```python
from build123d import *

# Parameters (mm, degrees)
SKETCH1_W           = 60
SKETCH1_H           = 35
BOSS_EXTRUDE1_DEPTH = 6.5
SKETCH2_W           = 50
SKETCH2_H           = 10
CUT_EXTRUDE1_DEPTH  = 70.765679241
FILLET1_R           = 10
CUT_EXTRUDE2_REACH  = 71.766
SKETCH3_R           = 2.5
CUT_EXTRUDE3_DEPTH  = 70.765679241
CUT_EXTRUDE4_DEPTH  = 70.765679241
FILLET6_R           = 2
FILLET7_R           = 2
FILLET8_R           = 2
FILLET9_R           = 2


with BuildPart() as part:
    # Sketch1 → Boss-Extrude1 (new body)
    with BuildSketch(Plane.XY):
        with Locations((30, 17.5)):
            Rectangle(SKETCH1_W, SKETCH1_H)
    extrude(amount=BOSS_EXTRUDE1_DEPTH)

    # Sketch2 → Cut-Extrude1 (cut, through all)
    with BuildSketch(Plane.XY.offset(6.5)):
        with Locations((25, 5)):
            Rectangle(SKETCH2_W, SKETCH2_H)
    extrude(amount=-CUT_EXTRUDE1_DEPTH, mode=Mode.SUBTRACT)

    # Fillet1
    fillet1_edges = [part.edges().sort_by_distance(p)[0] for p in [
        (0, 10, 3.25),
    ]]
    fillet(fillet1_edges, radius=FILLET1_R)

    # Sketch3 → Cut-Extrude2 (cut, up to next)
    with BuildSketch(Plane.XY.offset(6.5), mode=Mode.PRIVATE) as cut_extrude2_sk1:
        with Locations((10, 20)):
            Circle(SKETCH3_R)
    cut_extrude2_tool1 = extrude(cut_extrude2_sk1.sketch, amount=-CUT_EXTRUDE2_REACH, mode=Mode.PRIVATE) & part.part
    add(cut_extrude2_tool1.solids().sort_by_distance((10, 20, 6.5))[0], mode=Mode.SUBTRACT)

    # Sketch4 → Cut-Extrude3 (cut, through all)
    with BuildSketch(Plane.XY.offset(6.5)):
        Polygon((55, 0), (60, 16), (60, 0), align=None)
    extrude(amount=-CUT_EXTRUDE3_DEPTH, mode=Mode.SUBTRACT)

    # Sketch5 → Cut-Extrude4 (cut, through all)
    with BuildSketch(Plane.XY.offset(6.5)):
        Polygon((0, 35), (60, 16), (60, 35), align=None)
    extrude(amount=-CUT_EXTRUDE4_DEPTH, mode=Mode.SUBTRACT)

    # Fillet6
    fillet6_edges = [part.edges().sort_by_distance(p)[0] for p in [
        (50, 0, 3.25),
    ]]
    fillet(fillet6_edges, radius=FILLET6_R)

    # Fillet7
    fillet7_edges = [part.edges().sort_by_distance(p)[0] for p in [
        (55, 0, 3.25),
    ]]
    fillet(fillet7_edges, radius=FILLET7_R)

    # Fillet8
    fillet8_edges = [part.edges().sort_by_distance(p)[0] for p in [
        (60, 16, 3.25),
    ]]
    fillet(fillet8_edges, radius=FILLET8_R)

    # Fillet9
    fillet9_edges = [part.edges().sort_by_distance(p)[0] for p in [
        (0, 35, 3.25),
    ]]
    fillet(fillet9_edges, radius=FILLET9_R)


solid = part.part
```
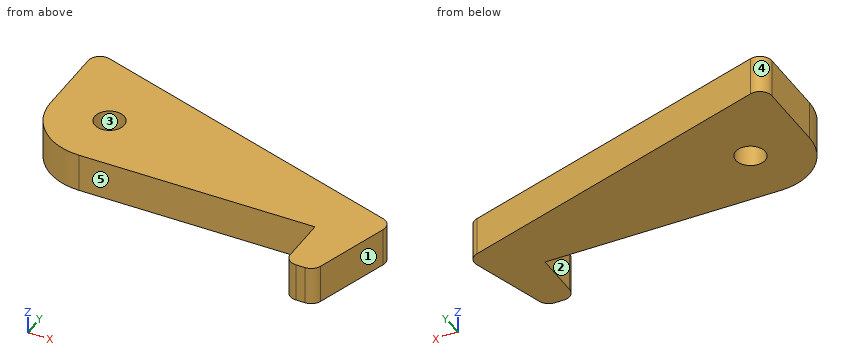
Check sheet for the modelled part. Datum: model origin and axes. Units: mm. Face numbers are marked on the shaded views. A direction names the side the tool comes from. Coordinates: 2 decimals unless noted, no trailing zeros. Write each loop counter-clockwise with the first axis right and the second up, starting at its lowest first coordinate (ties: lowest second). Pieces come first, ordered by that corner, then holes. Notation, with made-up numbers: M -32,13.5 L -5,13.5 A26 ccw -5,28.5 Z; hole C 26.25,-29.5 d10. An arc over 180 degrees is marked long. Use one line per item in the form item = value.
Item 1: Sectioned sample at D-D, the plane x = 25.5. Record the cut outline in (y, z) (3 decimals), and give its area (3 significant figures).
Answer below:
outline = M 10,0 L 26.925,0 L 26.925,6.5 L 10,6.5 Z
area = 110 mm^2
Item 2: Release check for a two-part mould opening along Y. For the marked faces 1, 2 and 3 record: pulls with the +Y half, pulls with the -Y half, needs draft (parallel to the pull), parting line crosses it, or undercut.
Answer below:
face_1 = pulls with the -Y half
face_2 = needs draft
face_3 = undercut
Item 3: Sectioned sample at A-A, the plane z = 1. Record the cut outline in (x, y).
Answer below:
outline = M 0,20 A10 ccw 10,10 L 50,10 L 50,2 A2 ccw 52,0 L 53.53,0 A2 ccw 55.44,1.4 L 59.41,14.1 A2 ccw 58.1,16.6 L 2.6,34.18 A2 ccw 0,32.27 Z; hole C 10,20 d5
Item 4: Material ranges on L1, parallel to Y at x = 10, z = 2.75; L2, parallel to Y at x = 53, z = 5; L3, parallel to Y at x = 32, z = 2.5, recorded low to high. Write a range as from..to.
Answer below:
L1 = 10..17.5, 22.5..31.83
L2 = 0..18.22
L3 = 10..24.87
Item 5: Sectioned sample at B-B, the plane x = 11. Record the cut outline in (y, z).
Answer below:
outline = M 10,0 L 17.71,0 L 17.71,6.5 L 10,6.5 Z; M 22.29,0 L 31.52,0 L 31.52,6.5 L 22.29,6.5 Z
Item 6: Sectioned sample at C-C, the plane y = 29.5. Record the cut outline in (x, z), and give its area (3 significant figures).
Answer below:
outline = M 0,0 L 17.37,0 L 17.37,6.5 L 0,6.5 Z
area = 113 mm^2
Item 7: Set-up check for the marked faces 4 and 5: record each of +Z, -Z, +X, -X, +Y, -Y from which the full face is reachable in a straight line by a thin tool's end or side.
Answer below:
face_4 = +Z, -Z, +Y
face_5 = +Z, -Z, -X, -Y
Item 8: Gauge pin test, flat ends, axial feed: pin 1 Ø4.5 at (x, y) = (10, 20) entering from -Z; pin 2 Ø1.5 at (x, z) = (44.5, 2) entering from -Y. Record the tip position at first contact, or that the pin passes through.
Answer below:
pin_1 = through
pin_2 = 10
